For this review, take the finished solid that the model builds, in its own axes (mm). A direction names the side the tool comes from. Give positions to 0.01 mm unless a question says otherwise; leave off trailing zeros. Write each loop counter-clockwise with the first axis right and the second up, starting at its lowest first coordinate (ties: lowest second). Pieces come first, ordered by that corner, then holes.
1) Wall thickness on line 1 along X through (y, z) = (1.25, -2.5); line 2 along Z through (x, y) = (17.5, 1.8); line 3 along X through (y, z) = (0.9, -60): over which ranges is each line inside the solid? List them lowest first.
2) Draft analysis for pull direction Z (two halves, no side actions). For faces 6 (the face through (-45.1, 0.99, -58.14)), 7 (the face through (-25.1, 1, -26.5)), 8 (the face through (0, 1, -17)), 9 (the face through (-24.024, 0.986, -29.508)), state which applies: pulls with the +Z half, pulls with the -Z half, needs draft (parallel to the pull), parting line crosses it, or undercut.
3) We need section A-A on z = -2.5. Give the boundary of the cut face in (x, y).
4) We need section C-C on z = -45. Give the boundary of the cut face in (x, y), and give its area (3 significant figures).
5) Machinability: for faces 1 (the face through (34.5, 1, -2.4)), 2 (the face through (-36, 1, -30)), 3 (the face through (-3, 1, -59)), 4 (the face through (-0.9, 0.99, -29.14)), 5 (the face through (-3.5, 1, -2.6)), which of the approach directions +Z, -Z, +X, -X, +Y, -Y give a long, thin tool a straight path to every point of the face, cutting with its end or side? Answer none if there is none.
6) For P1, Ø18, axis at x = 15.5, z = -17.5, coming from the +Y side; P2, Ø0.6, axis at x = 5, y = 1, coming from the -Z side; P3, Ø0.6, axis at x = -8.5, y = 1, coming from the +Z side, all flat-tipped, find the tip position at first contact; note any pin that passes through.
7) We need section D-D on y = 0.55. Give the number of separate pieces and of enclosed holes in the cut face, and give its area (3 significant figures).
8) We need section B-B on x = -38. Give the boundary of the cut face in (y, z).
from build123d import *

# Parameters (mm, degrees)
CROQUIS1_R              = 10
CROQUIS1_R_2            = 7.5
CROQUIS1_R_3            = 1.1
SALIENTE_EXTRUIR1_DEPTH = 2
CHAFL_N1_SIZE           = 1
CROQUIS2_R              = 1.25
CORTAR_EXTRUIR1_DEPTH   = 78.628925022


with BuildPart() as part:
    # Croquis1 → Saliente-Extruir1 (new body)
    with BuildSketch(Plane(origin=(0, 0, 0), x_dir=(1, 0, 0), z_dir=(0, 1, 0))):
        with BuildLine():
            Line((-43, 30), (-28.5, 30))
            ThreePointArc((-28.5, 30), (-27.792893219, 29.707106781), (-27.5, 29))
            ThreePointArc((-27.5, 29), (-25, 26.5), (-22.5, 29))
            ThreePointArc((-22.5, 29), (-22.207106781, 29.707106781), (-21.5, 30))
            Line((-21.5, 30), (-3, 30))
            ThreePointArc((-3, 30), (-0.878679656, 29.121320344), (0, 27))
            Line((0, 27), (0, 6))
            ThreePointArc((0, 6), (-0.292893219, 5.292893219), (-1, 5))
            ThreePointArc((-1, 5), (-3.5, 2.5), (-1, 0))
            Line((-1, 0), (0, 0))
            Line((0, 0), (31, 0))
            Line((31, 0), (32, 0))
            ThreePointArc((32, 0), (34.5, 2.5), (32, 5))
            ThreePointArc((32, 5), (31.292893219, 5.292893219), (31, 6))
            Line((31, 6), (31, 56))
            ThreePointArc((31, 56), (30.121320344, 58.121320344), (28, 59))
            Line((28, 59), (-34.5, 59))
            ThreePointArc((-34.5, 59), (-35.207106781, 59.292893219), (-35.5, 60))
            ThreePointArc((-35.5, 60), (-38, 62.5), (-40.5, 60))
            ThreePointArc((-40.5, 60), (-40.792893219, 59.292893219), (-41.5, 59))
            Line((-41.5, 59), (-43, 59))
            ThreePointArc((-43, 59), (-45.121320344, 58.121320344), (-46, 56))
            Line((-46, 56), (-46, 33))
            ThreePointArc((-46, 33), (-45.121320344, 30.878679656), (-43, 30))
        make_face()
        with Locations(Location((15.5, 17.5, 0), (0, 0, 270))):
            Circle(CROQUIS1_R, mode=Mode.SUBTRACT)
        with Locations(Location((16.5, 45, 0), (0, 0, 270))):
            Circle(CROQUIS1_R_2, mode=Mode.SUBTRACT)
        with Locations(Location((32, 2.5, 0), (0, 0, 270))):
            Circle(CROQUIS1_R_3, mode=Mode.SUBTRACT)
        with Locations(Location((-38, 60, 0), (0, 0, 270))):
            Circle(CROQUIS1_R_3, mode=Mode.SUBTRACT)
        with Locations(Location((-1, 2.5, 0), (0, 0, 90))):
            Circle(CROQUIS1_R_3, mode=Mode.SUBTRACT)
        with Locations(Location((-25, 29, 0), (0, 0, 90))):
            Circle(CROQUIS1_R_3, mode=Mode.SUBTRACT)
        with Locations(Location((28, 56, 0), (0, 0, 270))):
            Circle(CROQUIS1_R_3, mode=Mode.SUBTRACT)
    extrude(amount=SALIENTE_EXTRUIR1_DEPTH)

    # Chaflán1
    chafl_n1_edges = [part.edges().sort_by_distance(p)[0] for p in [
        (15.5, 2, -27.5),
        (16.5, 2, -52.5),
    ]]
    chamfer(chafl_n1_edges, length=CHAFL_N1_SIZE)

    # Croquis2 → Cortar-Extruir1 (cut, through all)
    with BuildSketch(Plane(origin=(0, 2, 0), x_dir=(1, 0, 0), z_dir=(0, 1, 0))):
        with Locations(Location((-34, 52.5, 0), (0, 0, 270))):
            Circle(CROQUIS2_R)
        with Locations(Location((-34, 36.5, 0), (0, 0, 270))):
            Circle(CROQUIS2_R)
    extrude(amount=-CORTAR_EXTRUIR1_DEPTH, mode=Mode.SUBTRACT)


solid = part.part
Results list:
1. line 1: x = -3.5 to -2.1, 0.1 to 30.9, 33.1 to 34.5
1. line 2: z = -59 to -53.24, -36.76 to -28.11, -6.89 to 0
1. line 3: x = -40.5 to -39.1, -36.9 to -35.5
2. face 6: pulls with the -Z half
2. face 7: pulls with the +Z half
2. face 8: undercut
2. face 9: undercut
3. outline: (-3.5, 0) - (-2.1, 0) - (-2.1, 2) - (-3.5, 2) - close; (0.1, 0) - (30.9, 0) - (30.9, 2) - (0.1, 2) - close; (33.1, 0) - (34.5, 0) - (34.5, 2) - (33.1, 2) - close
4. outline: (-46, 0) - (9, 0) - (9, 1) - (8, 2) - (-46, 2) - close; (24, 0) - (31, 0) - (31, 2) - (25, 2) - (24, 1) - close
4. area: 123 mm2
5. face 1: +X, +Y, -Y
5. face 2: +Z, -X, +Y, -Y
5. face 3: -Z, +X, +Y, -Y
5. face 4: +Y, -Y
5. face 5: -X, +Y, -Y
6. P1: passes through
6. P2: stops at z = -59
6. P3: stops at z = -30
7. separate pieces: 1
7. enclosed holes: 9
7. area: 2,700 mm2
8. outline: (0, -62.5) - (2, -62.5) - (2, -61.1) - (0, -61.1) - close; (0, -58.9) - (2, -58.9) - (2, -30) - (0, -30) - close
